```python
from build123d import *

# Parameters (mm, degrees)
F0_W     = 120
F0_H     = 120
F1_DEPTH = 30
F2_R     = 35
F2_R_2   = 25
F3_DEPTH = 25
F4_R     = 25
F5_DEPTH = 55.001
F6_R     = 5
F7_R     = 1.5
F8_T     = -2.5


with BuildPart() as f1:
    # F0 (on Front) → F1 (new body)
    with BuildSketch(Plane.XZ):
        Rectangle(F0_W, F0_H)
    extrude(amount=F1_DEPTH)

    # F2 (on face) → F3 (join)
    with BuildSketch(Plane.XZ.offset(30)):
        Circle(F2_R)
        Circle(F2_R_2, mode=Mode.SUBTRACT)
    extrude(amount=F3_DEPTH)

    # F4 (on face) → F5 (cut, through all)
    with BuildSketch(Plane(origin=(0, 0, 0), x_dir=(-1, 0, 0), z_dir=(0, 1, 0))):
        Circle(F4_R)
    extrude(amount=-F5_DEPTH, mode=Mode.SUBTRACT)

    # F6
    f6_edges = [f1.edges().sort_by_distance(p)[0] for p in [
        (60, -15, 60),
        (60, -15, -60),
        (60, -30, 0),
        (0, -30, -60),
        (-60, -30, 0),
        (0, -30, 60),
        (-60, -15, 60),
        (-60, -15, -60),
        (-35, -30, 0),
    ]]
    fillet(f6_edges, radius=F6_R)

    # F7
    f7_edges = [f1.edges().sort_by_distance(p)[0] for p in [
        (-35, -55, 0),
    ]]
    fillet(f7_edges, radius=F7_R)

    # F8
    f8_openings = [f1.faces().sort_by_distance(p)[0] for p in [
        (0, 0, 58.302944),
    ]]
    offset(amount=F8_T, openings=f8_openings)


solid = f1.part
```
Can you work these out from the model? Positions are in its coordinate system, mm. A direction names the side the tool comes from. Coordinates: 2 decimals unless noted, no trailing zeros. Write each loop counter-clockwise with the first axis right and the second up, starting at its lowest first coordinate (ties: lowest second). Pieces come first, ordered by that corner, then holes. Notation, with made-up numbers: (-39.75, 24) - (-35.75, 24) arc R23 ccw to (-35.75, 55) - close; hole circle Ø5 at (-32.5, 47.25). An arc over 180 degrees is marked (long way). Return JSON: item names as keys, results as strings.
Q1. Thinking about a two-plate mould opening in Z: for faces 1 (the cylindrical face through (59, -13, 58)), 2 (the flat face through (-1, -12, -57.5)), 3 (the flat face through (12.1, 0, -22.3)), which applies, +Z half, -Z half, draft (parallel to the pull), parting line (faces both ways), or undercut?
Computed values:
{"face 1": "+Z half", "face 2": "undercut", "face 3": "draft"}
Q2. I'm going to push flat-ended pins straight in: pin 1 Ø1.5 at (x, z) = (-24, 26.5) entering from +Y; pin 2 Ø12 at (x, z) = (42.5, -46.5) entering from +Y; pin 3 Ø6 at (x, y) = (-17.5, -36.5) entering from -Z. Where does each tip first touch, or does it pass through?
Computed values:
{"pin 1": "stops at y = -28.37", "pin 2": "stops at y = -27.5", "pin 3": "stops at z = -31.86"}
Q3. If we section it at C-C (y = -5): Please give me the cut outline in (x, z).
Computed values:
{"outline": "(-60, -55) arc R5 ccw to (-55, -60) - (55, -60) arc R5 ccw to (60, -55) - (60, 55) arc R5 ccw to (55, 60) - (-55, 60) arc R5 ccw to (-60, 55) - close; circle Ø55 at (0, 0); hole (-57.5, -55) arc R2.5 ccw to (-55, -57.5) - (55, -57.5) arc R2.5 ccw to (57.5, -55) - (57.5, 55) arc R2.5 ccw to (55, 57.5) - (-55, 57.5) arc R2.5 ccw to (-57.5, 55) - close; hole circle Ø50 at (0, 0)"}
Q4. Please list where these lines run through material, in increasing order: L1, parallel to Z at x = 0, y = -40; L2, parallel to Z at x = 1, y = -12; L3, parallel to X at y = -9, z = -19. Write a range as from..to.
Computed values:
{"L1": "z = -35..-32.5, -27.5..-25, 25..27.5, 32.5..35", "L2": "z = -60..-57.5, -27.48..-24.98, 24.98..27.48, 57.5..60", "L3": "x = -60..-57.5, -19.88..-16.25, 16.25..19.88, 57.5..60"}
Q5. On a 3-axis mill with a long thin cutter (end or side, diameter ignored), from which of +Z, -Z, +X, -X, +Y, -Y can I reach the whole of each face in a straight line? I mean faces 4 (the flat face through (-1, -12, 57.5)), 5 (the flat face through (-1, -12, -60)), 6 (the cylindrical face through (-28, -44, -21)). Say none if no direction works.
Computed values:
{"face 4": "+Y", "face 5": "-Z, +X, -X, +Y, -Y", "face 6": "-Y"}
Q6. If we section it at D-D (z = -42.5): Please give me the cut outline in (x, y).
Computed values:
{"outline": "(-60, -25) arc R5 ccw to (-55, -30) - (55, -30) arc R5 ccw to (60, -25) - (60, 0) - (57.5, 0) - (57.5, -25) arc R2.5 cw to (55, -27.5) - (-55, -27.5) arc R2.5 cw to (-57.5, -25) - (-57.5, 0) - (-60, 0) - close"}
